Model file for the job. Use its own axes, mm. Face numbers are marked on the shaded views. Coordinates: 2 decimals unless noted, no trailing zeros. Write each loop counter-clockwise with the first axis right and the second up, starting at its lowest first coordinate (ties: lowest second). Pieces come first, ordered by that corner, then holes. Notation, with made-up numbers: (73, 25.25) -> (127, 25.25) arc R13 ccw to (127, 41.25) -> close; hole circle Ø1 at (-25, -4.75). An arc over 180 degrees is marked (long way). Answer as a JSON object with one key per item and string values. Group by question number.
Autodesk Inventor part; units mm, degrees
ref_plane "YZ Plane" through (0, 0, 0) normal (1, 0, 0) x (0, 1, 0)
ref_plane "XZ Plane" through (0, 0, 0) normal (0, 1, 0) x (-1, 0, 0)
ref_plane "XY Plane" through (0, 0, 0) normal (0, 0, 1) x (1, 0, 0)
sketch "Sketch1" plane through (0, 0, 0) normal (0, 0, 1) x (1, 0, 0)
  circle A0 centre (0, 0) radius 9.165
  line L0 (0, 0) -> (-2.3778, 0) construction
  circle A1 centre (-20, 0) radius 9.165
  circle A2 centre (-40, 0) radius 9.165
  circle A3 centre (-60, 0) radius 9.165
  arc A4 (10.165, 0) -> (0, 10.165) centre (0, 0) ccw
  arc A5 (-60, 10.165) -> (-70.165, 0) centre (-60, 0) ccw
  line L1 (-60, 10.165) -> (0, 10.165)
  line L2 (-50.835, 0) -> (-49.165, 0)
  line L3 (-30.835, 0) -> (-29.165, 0)
  line L4 (-10.835, 0) -> (-9.165, 0)
  line L5 (-70.165, 0) -> (-69.165, 0)
  line L6 (9.165, 0) -> (10.165, 0)
  dimension "d0" = 18.33
  dimension "d3" = 20
  dimension "d8" = 1
  dimension "d9" = 1
extrude "Extrusion1" add sketch "Sketch1" along normal mid plane 10 contours A0 L4 A1 L3 A2 L2 A3 L5 A5 L1 A4 L6
properties part number "batteryspacer"
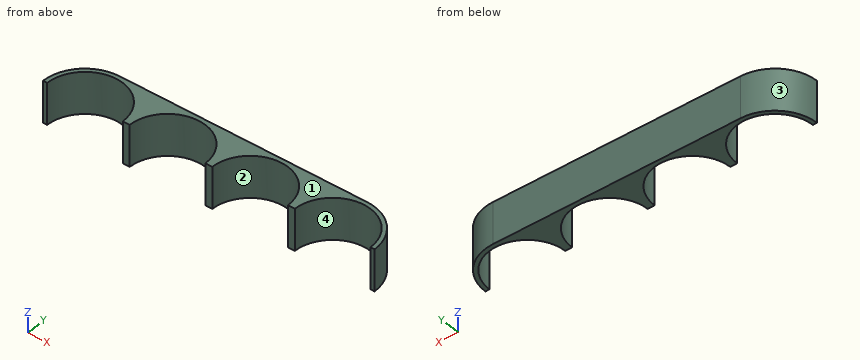
(1) Pull direction X, two halves, no side cores. Call the marked faces 1, 2, 3 and 4: released by +X, released by -X, zero draft, split by the parting line, or undercut.
(2) Cut at A-A on y = 5.25. List the corners of the cut face in (x, z), plus the area to 3 significant figures.
(3) Pin check, flat tips, straight feed: pin 1 (2 mm diameter, centred on y = 5.5, z = -2.5, fed in from +X); pin 2 (5 mm diameter, centred on x = -19.5, y = 6, fed in from +Z); pin 3 (1 mm diameter, centred on y = 5, z = -2, fed in from -X). Stop position of each tip, or through.
(4) Cut at D-D on x = -51.5. List the corners of the cut face in (y, z) (3 decimals).
(5) Cut at C-C on x = -20. List the corners of the cut face in (y, z) (3 decimals), plus the area to 3 significant figures.
(6) Cut at B-B on z = 0. List the corners of the cut face in (x, y) (3 decimals).
(7) Wall check: probe 1 along X at (y, z) = (8.5, 0.5); probe 2 along X at (y, z) = (7.75, -4.5); probe 3 along Y at (x, z) = (-27, 3.5) (3 decimals). Give the ranges that are in metal, low to high.
Results found:
{
 "1": {"face 1": "zero draft", "face 2": "undercut", "face 3": "released by -X", "face 4": "undercut"},
 "2": {"outline": "(-68.7, -5) -> (-67.51, -5) -> (-67.51, 5) -> (-68.7, 5) -> close; (-52.49, -5) -> (-47.51, -5) -> (-47.51, 5) -> (-52.49, 5) -> close; (-32.49, -5) -> (-27.51, -5) -> (-27.51, 5) -> (-32.49, 5) -> close; (-12.49, -5) -> (-7.51, -5) -> (-7.51, 5) -> (-12.49, 5) -> close; (7.51, -5) -> (8.7, -5) -> (8.7, 5) -> (7.51, 5) -> close", "area": "173 mm²"},
 "3": {"pin 1": "stops at x = 9.11", "pin 2": "passes through", "pin 3": "stops at x = -69.11"},
 "4": {"outline": "(3.427, -5) -> (10.165, -5) -> (10.165, 5) -> (3.427, 5) -> close"},
 "5": {"outline": "(9.165, -5) -> (10.165, -5) -> (10.165, 5) -> (9.165, 5) -> close", "area": "10.0 mm²"},
 "6": {"outline": "(-70.165, 0) -> (-69.165, 0) arc R9.165 cw to (-50.835, 0) -> (-49.165, 0) arc R9.165 cw to (-30.835, 0) -> (-29.165, 0) arc R9.165 cw to (-10.835, 0) -> (-9.165, 0) arc R9.165 cw to (9.165, 0) -> (10.165, 0) arc R10.165 ccw to (0, 10.165) -> (-60, 10.165) arc R10.165 ccw to start"},
 "7": {"probe 1": "x = -65.57 to -63.43, -56.57 to -43.43, -36.57 to -23.43, -16.57 to -3.43, 3.43 to 5.57", "probe 2": "x = -66.58 to -64.89, -55.11 to -44.89, -35.11 to -24.89, -15.11 to -4.89, 4.89 to 6.58", "probe 3": "y = 5.916 to 10.165"}
}
